Autodesk Inventor part; units mm, degrees
ref_plane "YZ Plane" through (0, 0, 0) normal (1, 0, 0) x (0, 1, 0)
ref_plane "XZ Plane" through (0, 0, 0) normal (0, 1, 0) x (-1, 0, 0)
ref_plane "XY Plane" through (0, 0, 0) normal (0, 0, 1) x (1, 0, 0)
sketch "Sketch1" plane through (0, 0, 0) normal (0, 1, 0) x (-1, 0, 0)
  line L0 (0, 0) -> (100, 0)
  line L1 (100, 0) -> (100, -100)
  line L2 (100, -100) -> (0, -100)
  line L3 (0, -100) -> (0, 0)
  line L4 (100, 0) -> (0, -100)
  line L5 (100, -100) -> (0, 0)
  line L6 (-15, 35) -> (115, 35)
  line L7 (115, 35) -> (115, -135)
  line L8 (115, -135) -> (-15, -135)
  line L9 (-15, -135) -> (-15, 35)
  line L10 (-15, 35) -> (115, -135) construction
  line L11 (115, 35) -> (-15, -135) construction
  line L12 (115, 35) -> (115, 15)
  line L13 (115, 15) -> (75, 15)
  line L14 (75, 15) -> (75, 35)
  line L15 (-15, 35) -> (-15, 15)
  line L16 (-15, 15) -> (25, 15)
  line L17 (25, 15) -> (25, 35)
  line L18 (75, 15) -> (67.5, 15)
  line L19 (67.5, 15) -> (67.5, 35)
  line L20 (25, 15) -> (32.5, 15)
  line L21 (32.5, 15) -> (32.5, 35)
  line L22 (32.5, 35) -> (-15, 15)
  line L23 (67.5, 35) -> (115, 15)
  line L24 (115, -135) -> (115, -115)
  line L25 (115, -115) -> (67.5, -115)
  line L26 (67.5, -115) -> (67.5, -135)
  line L27 (-15, -135) -> (-15, -115)
  line L28 (-15, -115) -> (32.5, -115)
  line L29 (32.5, -115) -> (32.5, -135)
  line L30 (115, -115) -> (67.5, -135)
  line L31 (-15, -115) -> (32.5, -135)
  line L32 (100, 0) -> (100, -10)
  line L33 (100, -10) -> (90, -10)
  line L34 (90, -10) -> (90, 0)
  line L35 (100, -100) -> (100, -90)
  line L36 (100, -90) -> (90, -90)
  line L37 (90, -90) -> (90, -100)
  line L38 (0, -100) -> (10, -100)
  line L39 (10, -100) -> (10, -90)
  line L40 (10, -90) -> (0, -90)
  line L41 (0, 0) -> (10, 0)
  line L42 (10, 0) -> (10, -10)
  line L43 (0, -10) -> (10, -10)
  line L44 (90, 0) -> (100, -10)
  line L45 (100, -90) -> (90, -100)
  line L46 (0, -90) -> (10, -100)
  line L47 (10, 0) -> (0, -10)
  line L48 (50, -135) -> (50, -130)
  line L49 (41, -130) -> (59, -130)
  line L50 (59, -130) -> (59, -106)
  line L51 (59, -106) -> (41, -106)
  line L52 (41, -106) -> (41, -130)
  line L53 (50, 35) -> (50, 30)
  line L54 (41, 30) -> (59, 30)
  line L55 (59, 30) -> (59, 6)
  line L56 (59, 6) -> (41, 6)
  line L57 (41, 6) -> (41, 30)
  point P0 (50, -50)
  dimension "d0" = 100
  dimension "d1" = 100
  dimension "d4" = 130
  dimension "d5" = 170
  dimension "d6" = 20
  dimension "d7" = 40
  dimension "d8" = 40
  dimension "d10" = 7.5
  dimension "d11" = 7.5
  dimension "d12" = 20
  dimension "d13" = 47.5
  dimension "d14" = 10
  dimension "d15" = 10
  dimension "d16" = 10
  dimension "d17" = 10
  dimension "d22" = 5
  dimension "d23" = 18
  dimension "d24" = 24
  dimension "d25" = 5
  dimension "d26" = 18
  dimension "d27" = 24
extrude "Extrusion1" add sketch "Sketch1" against normal blind 5 contours L5 L47 L3 | L0 L47 L5 | L0 L4 L44 | L46 L4 L3 | L1 L44 L4 | L4 L46 L2 | L1 L5 L45 | L5 L2 L45 | L49 L52 L51 L50 | L54 L55 L56 L57 | L16 L20 L21 L6 L19 L18 L13 L7 L25 L26 L8 L29 L28 L9 | L22 L17 L16 | L21 L20 L17 L22 | L28 L29 L31 | L23 L14 L18 L19 | L23 L13 L14 | L26 L25 L30
extrude "Extrusion2" add sketch "Sketch1" along normal blind 2 contours L49 L52 L51 L50 | L54 L55 L56 L57 | L16 L20 L21 L6 L19 L18 L13 L7 L25 L26 L8 L29 L28 L9 | L22 L17 L16 | L21 L20 L17 L22 | L28 L29 L31 | L23 L14 L18 L19 | L23 L13 L14 | L26 L25 L30
hole "Hole1" at (-59, 0, 30) at (-59, 0, 6) at (-41, 0, 30) at (-41, 0, 6) at (-59, 0, -130) at (-41, 0, -130) at (-41, 0, -106) at (-59, 0, -106) direction (0, -1, 0) diameter 3.4 end through all both
properties part number "BedHousingFrame"
Input: part model. Units: mm. Frame: model coordinates. A direction names the side the tool comes from. Give positions to 0.01 mm unless a question says otherwise; leave off trailing zeros. Order: outer loops, then holes, each group sorted by start corner. A loop starts at its lowest first (then second) coordinate and runs counter-clockwise, first axis right, second up. Notation, with made-up numbers: (75, 8) - (107, 8) arc R19 cw to (107, 23) - close; hole circle Ø8 at (22.5, 14). An arc over 180 degrees is marked (long way). Put each result on its own line as item: value.
Item 1: Section query A-A, the plane z = -64. Return loops of the section in (x, y).
Found:
outline: (-115, -5) - (-100, -5) - (-100, 2) - (-115, 2) - close; (0, -5) - (15, -5) - (15, 2) - (0, 2) - close
Item 2: Section query B-B, the plane x = -64. Return loops of the section in (y, z).
Found:
outline: (-5, -135) - (2, -135) - (2, -100) - (-5, -100) - close; (-5, 0) - (2, 0) - (2, 35) - (-5, 35) - close
Item 3: Section query C-C, the plane y = -3.5. Count the separate pieces of the cut face and the enclosed holes in it, then the cut area to 3 significant figures.
Found:
separate pieces: 1
enclosed holes: 9
area: 10,300 mm^2
Item 4: Ray query, L1, parallel to Z at x = -59, y = -1.75; L2, parallel to X at y = -2.25, z = 6; L3, parallel to X at y = -4, z = -17.5. Return the intervals inside material, ascending. Write a range as from..to.
Found:
L1: z = -135..-131.7, -128.3..-107.7, -104.3..-100, 0..4.3, 7.7..28.3, 31.7..35
L2: x = -115..-60.7, -57.3..-42.7, -39.3..15
L3: x = -115..-100, 0..15
Item 5: Contact query for flat-ended pins moving along their axis: pin 1 (2 mm diameter, centred on x = -68, y = -2, fed in from -Z); pin 2 (5 mm diameter, centred on x = -6, z = -5.5, fed in from +Y); pin 3 (1.5 mm diameter, centred on x = -10, y = -1, fed in from -Z); pin 4 (4 mm diameter, centred on x = -17.5, y = -2.5, fed in from -Z). Output: stop coordinate, or through.
Found:
pin 1: stops at z = -135
pin 2: stops at y = 0
pin 3: stops at z = -125.84
pin 4: stops at z = -129.53
Item 6: Draft query along Z for faces 1 (the flat face through (-51, -1, -100)), 2 (the flat face through (-90.92, -1.45, 25.14)), 3 (the flat face through (-115, -1, -49)), 4 (the flat face through (-4, 0, -4)). Return one class per face: +Z half, -Z half, draft (parallel to the pull), parting line (faces both ways), or undercut.
Found:
face 1: undercut
face 2: +Z half
face 3: draft
face 4: undercut
Item 7: Section query D-D, the plane z = -98. Return loops of the section in (x, y), then the cut area to 3 significant figures.
Found:
outline: (-115, -5) - (-92, -5) - (-92, 0) - (-100, 0) - (-100, 2) - (-115, 2) - close; (-8, -5) - (15, -5) - (15, 2) - (0, 2) - (0, 0) - (-8, 0) - close
area: 290 mm^2
Item 8: Access query for faces 5 (the flat face through (-91.58, -1.45, -124.86)), 6 (the flat face through (-3, 0, -97)), 7 (the flat face through (-95, -2, -95)). Directions: +Z, -Z, +X, -X, +Y, -Y. A direction counts if a zero-diameter tool reaches every point of the face in a straight line with its end or side. Return the directions, or none.
Found:
face 5: -Z, -X, +Y, -Y
face 6: +Y
face 7: +Y, -Y
